Work out the finished part from the listing and answer in its coordinate system (mm). A direction names the side the tool comes from. Coordinates: 2 decimals unless noted, no trailing zeros. Loops run counter-clockwise (first coordinate to the right, second up) from the corner with the lowest first, then second, coordinate; pieces in that order, holes last. Notation, with made-up numbers: (-23, 51.5) - (-17, 51.5) arc R24 cw to (-17, 71.5) - close; hole circle Ø5 at (52, 61.25). An arc over 180 degrees is marked (long way). Write each question's results on one line, items separated by ' | '. Start each with the question number.
1. A cutting plane is placed at A-A on z = 0. Determine the outline of the cut face in (x, y) (3 decimals), then the cut area to 3 significant figures.
2. Find the intervals of material crossed by line 1 along X through (y, z) = (4.15, 0) (3 decimals); line 2 along X through (y, z) = (2.55, 0); line 3 along Y through (x, z) = (25.5, 2.5), in increasing order. Write a range as [from, to].
3. Determine the mould class of faces 1 (the flat face through (11, 3, -5)), 2 (the flat face through (12, 3, 5)), 3 (the cylindrical face through (20.943, 4.768, 0.27)) for opening direction Z: released by +Z, released by -Z, zero draft, split by the parting line, or undercut.
4. A cutting plane is placed at C-C on x = -3. Determine the outline of the cut face in (y, z).
5. A cutting plane is placed at D-D on x = 24. Determine the outline of the cut face in (y, z), then the cut area to 3 significant figures.
6. Each of these flat-tipped pins is pushed along its axis until it touches: P1, Ø3.5, axis at x = 23, z = 0, coming from the -Y side; P2, Ø2, axis at x = 23.5, z = 1, coming from the -Y side. Where does it stop, or does it pass through?
7. Which of the six approach directions +Z, -Z, +X, -X, +Y, -Y give full straight-line access (tool end or side, diameter ignored) to faces 4 (the cylindrical face through (-5, 3, 0)), 5 (the flat face through (25, 3.5, -2))?
8. A cutting plane is placed at B-B on y = 4.6. Determine the outline of the cut face in (x, z) (3 decimals), then the cut area to 3 significant figures.
from build123d import *

# Parameters (mm, degrees)
EXTRUDE_1_DEPTH = 6


with BuildPart() as part:
    # 草图1 → 凸台-拉伸1 (new body)
    with BuildSketch(Plane(origin=(0, 0, 0), x_dir=(1, 0, 0), z_dir=(0, 1, 0))):
        with BuildLine():
            Line((0, 5), (23, 5))
            ThreePointArc((23, 5), (28, 0), (23, -5))
            Line((23, -5), (0, -5))
            ThreePointArc((0, -5), (-5, 0), (0, 5))
        make_face()
    extrude(amount=EXTRUDE_1_DEPTH)

    # 草图2 → 切除-旋转1 (revolve, cut)
    with BuildSketch(Plane.XY, mode=Mode.PRIVATE) as cut_revolve_1_sk:
        Polygon((0, 0), (-3.75, 0), (-3.75, 3.5), (-2.075, 3.5), (-2.075, 6), (0, 6), align=None)
    revolve(cut_revolve_1_sk.sketch.rotate(Axis((0, 6, 0), (0, -1, 0)), 270), axis=Axis((0, 6, 0), (0, -1, 0)), mode=Mode.SUBTRACT)

    # 草图3 → 切除-旋转2 (revolve, cut)
    with BuildSketch(Plane.XY, mode=Mode.PRIVATE) as cut_revolve_2_sk:
        Polygon((23, 0), (19.25, 0), (19.25, 3.5), (20.925, 3.5), (20.925, 6), (23, 6), align=None)
    revolve(cut_revolve_2_sk.sketch.rotate(Axis((23, 0, 0), (0, 1, 0)), 270), axis=Axis((23, 0, 0), (0, 1, 0)), mode=Mode.SUBTRACT)


solid = part.part
Values:
1) outline: (-5, 0) - (-3.75, 0) - (-3.75, 3.5) - (-2.075, 3.5) - (-2.075, 6) - (-5, 6) - close; (2.075, 3.5) - (3.75, 3.5) - (3.75, 0) - (19.25, 0) - (19.25, 3.5) - (20.925, 3.5) - (20.925, 6) - (2.075, 6) - close; (25.075, 3.5) - (26.75, 3.5) - (26.75, 0) - (28, 0) - (28, 6) - (25.075, 6) - close | area: 125 mm^2
2) line 1: [-5, -2.075], [2.075, 20.925], [25.075, 28] | line 2: [-5, -3.75], [3.75, 19.25], [26.75, 28] | line 3: [3.5, 6]
3) face 1: released by -Z | face 2: released by +Z | face 3: undercut
4) outline: (0, -4) - (6, -4) - (6, 4) - (0, 4) - (0, 2.25) - (3.5, 2.25) - (3.5, -2.25) - (0, -2.25) - close
5) outline: (0, -4.9) - (6, -4.9) - (6, -1.82) - (3.5, -1.82) - (3.5, -3.61) - (0, -3.61) - close; (0, 3.61) - (3.5, 3.61) - (3.5, 1.82) - (6, 1.82) - (6, 4.9) - (0, 4.9) - close | area: 24.4 mm^2
6) P1: through | P2: y = 3.5
7) face 4: -X, +Y, -Y | face 5: -Y
8) outline: (0, -5) - (23, -5) arc R5 ccw to (23, 5) - (0, 5) arc R5 ccw to start; hole circle Ø4.15 at (0, 0); hole circle Ø4.15 at (23, 0) | area: 281 mm^2
